from build123d import *

# Parameters (mm, degrees)
SKETCH1_R           = 2.51
BOSS_EXTRUDE1_DEPTH = 5
SKETCH2_R           = 6.25
SKETCH2_R_2         = 4.25
BOSS_EXTRUDE2_DEPTH = 7.5
SKETCH2_3_R         = 4.25
CUT_EXTRUDE1_DEPTH  = 47.703854396
SKETCH1_3_W         = 20
SKETCH1_3_H         = 10
BOSS_EXTRUDE3_DEPTH = 20
SKETCH3_W           = 17.5
SKETCH3_H           = 6.5
CUT_EXTRUDE2_DEPTH  = 17.5
CUT_EXTRUDE3_REACH  = 59.663
SKETCH4_R           = 2.5


with BuildPart() as part:
    # Sketch1 → Boss-Extrude1 (new body)
    with BuildSketch(Plane(origin=(0, 0, 0), x_dir=(1, 0, 0), z_dir=(0, 1, 0))):
        with BuildLine():
            Line((2.51, -9.999999226), (45, -9.999999226))
            Line((45, -9.999999226), (45, 10.000000774))
            Line((45, 10.000000774), (2.51, 10.000000774))
            ThreePointArc((2.51, 10.000000774), (0, 7.490000774), (-2.51, 10.000000774))
            Line((-2.51, 10.000000774), (-45, 10.000000774))
            Line((-45, 10.000000774), (-45, -9.999999226))
            Line((-45, -9.999999226), (-2.51, -9.999999226))
            ThreePointArc((-2.51, -9.999999226), (0, -7.489999226), (2.51, -9.999999226))
        make_face()
        with Locations(Location((-10, 7.74e-07, 0), (0, 0, 270))):
            Circle(SKETCH1_R, mode=Mode.SUBTRACT)
        with Locations(Location((0, 7.74e-07, 0), (0, 0, 270))):
            Circle(SKETCH1_R, mode=Mode.SUBTRACT)
        with Locations(Location((10, 7.74e-07, 0), (0, 0, 270))):
            Circle(SKETCH1_R, mode=Mode.SUBTRACT)
    extrude(amount=BOSS_EXTRUDE1_DEPTH)

    # Sketch2 → Boss-Extrude2 (add)
    # profile 1 of 2: a face of its own
    with BuildSketch(Plane(origin=(0, 5, 0), x_dir=(1, 0, 0), z_dir=(0, 1, 0))):
        with Locations(Location((-30, 0, 0), (0, 0, 270))):
            Circle(SKETCH2_R)
        with Locations(Location((-30, 0, 0), (0, 0, 270))):
            Circle(SKETCH2_R_2, mode=Mode.SUBTRACT)
    # profile 2 of 2: a face of its own
    with BuildSketch(Plane(origin=(0, 5, 0), x_dir=(1, 0, 0), z_dir=(0, 1, 0))):
        with Locations(Location((30, 0, 0), (0, 0, 270))):
            Circle(SKETCH2_R)
        with Locations(Location((30, 0, 0), (0, 0, 270))):
            Circle(SKETCH2_R_2, mode=Mode.SUBTRACT)
    extrude(amount=BOSS_EXTRUDE2_DEPTH)

    # Sketch2<3> → Cut-Extrude1 (cut, through all)
    with BuildSketch(Plane(origin=(0, 5, 0), x_dir=(1, 0, 0), z_dir=(0, 1, 0))):
        with Locations(Location((-30, 0, 0), (0, 0, 270))):
            Circle(SKETCH2_3_R)
        with Locations(Location((30, 0, 0), (0, 0, 270))):
            Circle(SKETCH2_3_R)
    extrude(amount=-CUT_EXTRUDE1_DEPTH, mode=Mode.SUBTRACT)

    # Sketch1<3> → Boss-Extrude3 (add)
    with BuildSketch(Plane(origin=(0, 0, 0), x_dir=(1, 0, 0), z_dir=(0, 1, 0))):
        with Locations((35, -14.999999226)):
            Rectangle(SKETCH1_3_W, SKETCH1_3_H)
        with Locations((-35, -14.999999226)):
            Rectangle(SKETCH1_3_W, SKETCH1_3_H)
    extrude(amount=BOSS_EXTRUDE3_DEPTH)

    # Sketch3 → Cut-Extrude2 (cut)
    with BuildSketch(Plane(origin=(0, 20, 0), x_dir=(1, 0, 0), z_dir=(0, 1, 0))):
        with Locations((36.25, -14.999999226)):
            Rectangle(SKETCH3_W, SKETCH3_H)
        with Locations((-36.25, -14.999999226)):
            Rectangle(SKETCH3_W, SKETCH3_H)
    extrude(amount=-CUT_EXTRUDE2_DEPTH, mode=Mode.SUBTRACT)

    # Cut-Extrude3: up to this face of the body (flat: up to its plane)
    cut_extrude3_end = Plane(part.part.faces().sort_by_distance((35, 12.5, 9.999999226))[0])
    # Sketch4 → Cut-Extrude3 (cut, up to the picked face)
    with BuildSketch(Plane.XY.offset(19.999999226), mode=Mode.PRIVATE) as cut_extrude3_sk1:
        with Locations((37.5, 12.5)):
            Circle(SKETCH4_R)
    cut_extrude3_tool1 = split(extrude(cut_extrude3_sk1.sketch, amount=-CUT_EXTRUDE3_REACH, mode=Mode.PRIVATE), bisect_by=cut_extrude3_end, keep=Keep.BOTH, mode=Mode.PRIVATE)
    # Sketch4 → Cut-Extrude3 (cut, up to the picked face)
    with BuildSketch(Plane.XY.offset(19.999999226), mode=Mode.PRIVATE) as cut_extrude3_sk2:
        with Locations((-37.5, 12.5)):
            Circle(SKETCH4_R)
    cut_extrude3_tool2 = split(extrude(cut_extrude3_sk2.sketch, amount=-CUT_EXTRUDE3_REACH, mode=Mode.PRIVATE), bisect_by=cut_extrude3_end, keep=Keep.BOTH, mode=Mode.PRIVATE)
    add(cut_extrude3_tool1.solids().sort_by(Axis((37.5, 12.5, 19.999999), (0, 0, -1)))[0], mode=Mode.SUBTRACT)
    add(cut_extrude3_tool2.solids().sort_by(Axis((-37.5, 12.5, 19.999999), (0, 0, -1)))[0], mode=Mode.SUBTRACT)


solid = part.part
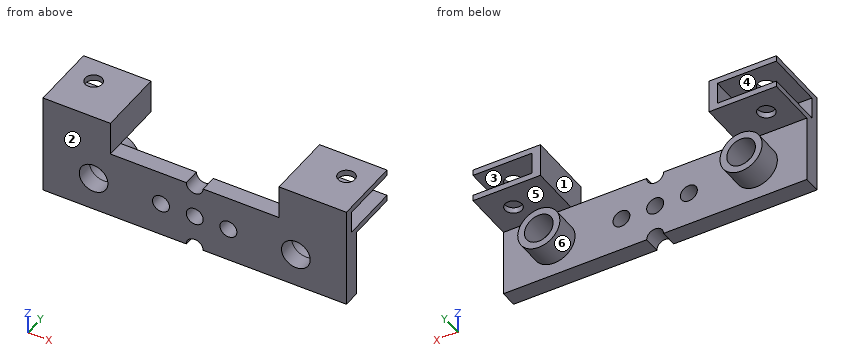
Could you check a few things on this model? Use its own coordinates, in mm. Face numbers are marked on the shaded views. A direction names the side the tool comes from. Give positions to 0.01 mm unless a question says otherwise; leave off trailing zeros. Order: outer loops, then holes, each group sorted by start corner. A loop starts at its lowest first (then second) coordinate and runs counter-clockwise, first axis right, second up. Notation, with made-up numbers: (17.25, 40) -> (39.25, 40) arc R20 cw to (39.25, 51) -> close; hole circle Ø11 at (-26.5, -16.75). An arc over 180 degrees is marked (long way). Answer in a Markdown table with one row per item. Add a question column.
Item 1: Please list where these lines run through material, in increasing order: probe 1 along X at (y, z) = (3, 0); probe 2 along Z at (x, y) = (-35, 13.75); probe 3 along X at (y, z) = (16.75, 14).
Item 2: Imagine slicing it at D-D (z = 13.25). List the corners of the cut face in (x, y) for me, and give its area (4 significant figures).
Item 3: Imagine slicing it at A-A (z = 0). Count the separate pieces of the cut face and the enclosed holes in it, and give its area (3 significant figures).
Item 4: I'm going to push flat-ended pins straight in: P1, Ø8, axis at x = 3, y = 5.5, coming from the +Z side; P2, Ø4.5, axis at x = 37.5, y = 12.5, coming from the -Z side; P3, Ø2, axis at x = 33, z = 14, coming from the +Y side; P4, Ø7.5, axis at x = 30, z = 0, coming from the -Y side. Where does each tip first touch, or does it pass through?
Item 5: For the marked faces 3, 4, 5 and 6, which set-ups out of +Z, -Z, +X, -X, +Y, -Y let a thin tool reach every point of the face, with its end or its side?
Item 6: Imagine slicing it at C-C (y = 6.5). List the corners of the cut face in (x, z) for me.
Item 7: Imagine slicing it at B-B (x = -37.5). List the corners of the cut face in (y, z) for me, and give its area (3 significant figures).
Item 8: We'd pull the mould along X, two halves only. Please class the marked faces 1 and 2: pulls with the +X half, pulls with the -X half, needs draft (parallel to the pull), parting line crosses it, or undercut.
Result:
| question | item | result |
|---|---|---|
| 1 | probe 1 | -45 to -34.25, -25.75 to -12.51, -7.49 to -2.51, 2.51 to 7.49, 12.51 to 25.75, 34.25 to 45 |
| 1 | probe 2 | 10 to 11.75, 18.25 to 20 |
| 1 | probe 3 | -27.5 to -25, 25 to 27.5 |
| 2 | outline | (-45, 0) -> (-25, 0) -> (-25, 20) -> (-27.5, 20) -> (-27.5, 2.5) -> (-45, 2.5) -> close; (25, 0) -> (45, 0) -> (45, 2.5) -> (27.5, 2.5) -> (27.5, 20) -> (25, 20) -> close |
| 2 | area | 187.5 mm2 |
| 3 | separate pieces | 6 |
| 3 | enclosed holes | 0 |
| 3 | area | 350 mm2 |
| 4 | P1 | z = 10 |
| 4 | P2 | z = -3.39 |
| 4 | P3 | y = 2.5 |
| 4 | P4 | through |
| 5 | face 3 | +X, +Y |
| 5 | face 4 | -X, +Y |
| 5 | face 5 | +X, -X, +Y |
| 5 | face 6 | +Y |
| 6 | outline | (-45, 10) -> (-25, 10) -> (-25, 20) -> (-45, 20) -> (-45, 18.25) -> (-27.5, 18.25) -> (-27.5, 11.75) -> (-45, 11.75) -> close; circle Ø12.5 at (-30, 0); circle Ø12.5 at (30, 0); (25, 10) -> (45, 10) -> (45, 11.75) -> (27.5, 11.75) -> (27.5, 18.25) -> (45, 18.25) -> (45, 20) -> (25, 20) -> close; hole circle Ø8.5 at (-30, 0); hole circle Ø8.5 at (30, 0) |
| 7 | outline | (0, -10) -> (5, -10) -> (5, 10) -> (10, 10) -> (10, 11.75) -> (2.5, 11.75) -> (2.5, 18.25) -> (10, 18.25) -> (10, 20) -> (0, 20) -> close; (15, 10) -> (20, 10) -> (20, 11.75) -> (15, 11.75) -> close; (15, 18.25) -> (20, 18.25) -> (20, 20) -> (15, 20) -> close |
| 7 | area | 169 mm2 |
| 8 | face 1 | undercut |
| 8 | face 2 | needs draft |
